```python
from build123d import *

# Parameters (mm, degrees)
SKETCH1_W               = 508
SKETCH1_H               = 228.6
BOSS_EXTRUDE1_DEPTH     = 254
SKETCH2_W               = 127
SKETCH2_H               = 93.154290468
CUT_EXTRUDE1_DEPTH      = 509
CUT_EXTRUDE2_DEPTH      = 254
SKETCH7_W               = 127
SKETCH7_H               = 101.6
CUT_EXTRUDE3_DEPTH      = 127
CUT_EXTRUDE5_DEPTH      = 127
CUT_EXTRUDE5_DEPTH_BACK = 0.254
SKETCH24_W              = 127
SKETCH24_H              = 101.6
BOSS_EXTRUDE3_DEPTH     = 63.5
CUT_EXTRUDE7_DEPTH      = 315.976
SKETCH27_R              = 6.604
CUT_EXTRUDE8_DEPTH      = 315.976


with BuildPart() as part:
    # Sketch1 → Boss-Extrude1 (new body)
    with BuildSketch(Plane.XY):
        Rectangle(SKETCH1_W, SKETCH1_H)
    extrude(amount=BOSS_EXTRUDE1_DEPTH)

    # Sketch2 → Cut-Extrude1 (cut, through all)
    with BuildSketch(Plane.ZY.offset(254)):
        with Locations((127, 67.722854766)):
            Rectangle(SKETCH2_W, SKETCH2_H)
    extrude(amount=-CUT_EXTRUDE1_DEPTH, mode=Mode.SUBTRACT)

    # Sketch5 → Cut-Extrude2 (cut)
    with BuildSketch(Plane.XY.offset(254)):
        Polygon((-254, 0), (-254, -114.3), (127, -114.3), (-63.5, 0), align=None)
    extrude(amount=-CUT_EXTRUDE2_DEPTH, mode=Mode.SUBTRACT)

    # Sketch7 → Cut-Extrude3 (cut)
    with BuildSketch(Plane(origin=(254, 0, 0), x_dir=(0, 0, -1), z_dir=(1, 0, 0))):
        with Locations((-127, -29.654290468)):
            Rectangle(SKETCH7_W, SKETCH7_H)
    extrude(amount=-CUT_EXTRUDE3_DEPTH, mode=Mode.SUBTRACT)

    # Sketch20 → Cut-Extrude5 (cut, two sides)
    with BuildSketch(Plane(origin=(0, 0, 190.5), x_dir=(-1, 0, 0), z_dir=(0, 0, -1))) as cut_extrude5_sk:
        Polygon((-127, 21.145709532), (39.624, 21.145709532), (-127, -80.454290468), align=None)
    extrude(amount=CUT_EXTRUDE5_DEPTH, mode=Mode.SUBTRACT)
    extrude(cut_extrude5_sk.sketch, amount=-CUT_EXTRUDE5_DEPTH_BACK, mode=Mode.SUBTRACT)

    # Sketch24 → Boss-Extrude3 (add)
    with BuildSketch(Plane(origin=(254, 0, 0), x_dir=(0, 0, -1), z_dir=(1, 0, 0))):
        with Locations((-127, -29.654290468)):
            Rectangle(SKETCH24_W, SKETCH24_H)
    extrude(amount=-BOSS_EXTRUDE3_DEPTH)

    # Sketch26 → Cut-Extrude7 (cut)
    with BuildSketch(Plane.XY.offset(254)):
        Polygon((254, 114.3), (-63.5, 114.3), (254, 0), align=None)
    extrude(amount=-CUT_EXTRUDE7_DEPTH, mode=Mode.SUBTRACT)

    # Sketch27 → Cut-Extrude8 (cut)
    with BuildSketch(Plane.XY.offset(254)):
        with Locations((-203.2, 57.15)):
            Circle(SKETCH27_R)
    extrude(amount=-CUT_EXTRUDE8_DEPTH, mode=Mode.SUBTRACT)


solid = part.part
```
Could you check a few things on this model? Use its own coordinates, in mm. A direction names the side the tool comes from. Round coordinates to 2 decimals unless told otherwise and drop trailing zeros. Loops run counter-clockwise (first coordinate to the right, second up) from the corner with the lowest first, then second, coordinate; pieces in that order, holes last.
Q1. For P1, Ø12, axis at y = -7.5, z = 166, coming from the -X side; P2, Ø2, axis at x = 82.5, z = 225, coming from the +Y side; P3, Ø12, axis at x = 57, y = -9, coming from the -Z side; P4, Ø5, axis at x = 193, z = 131.5, coming from the +Y side, each with a flat end and sliding along its axis, tell me the tip position at first contact or that it passes through.
Q2. Please list where these lines run through material, in increasing order: L1, parallel to Z at x = -158, y = 39; L2, parallel to Y at x = -203.2, z = 232.5; L3, parallel to Y at x = 155.5, z = 114.
Q3. I want a section at A-A (x = -203.2). Write out the boundary of the cut face in (y, z).
Q4. I want a section at D-D (y = -40). Write out the boundary of the cut face in (x, z), and give its area (3 significant figures).
Q5. Thinking about a two-plate mould opening in X: for faces 1 (the flat face through (-160, 114.3, 31)), 2 (the flat face through (198.86, 19.85, 128.78)), 3 (the flat face through (33.08, -57.95, 128.78)), 4 (the flat face through (159, -80.454, 128)), which applies, pulls with the +X half, pulls with the -X half, needs draft (parallel to the pull), parting line crosses it, or undercut?
Q6. I want a section at B-B (z = 72.5). Write out the boundary of the cut face in (x, y).
Q7. I want a section at C-C (y = 57.15). Write out the boundary of the cut face in (x, z).
Q8. On a 3-axis mill with a long thin cutter (end or side, diameter ignored), from which of +Z, -Z, +X, -X, +Y, -Y can I reach the whole of each face in a straight line? I mean faces 5 (the flat face through (-148, 21.146, 126)), 6 (the flat face through (-157, 0, 129)), 7 (the flat face through (190.5, -29, 128)). Say none if no direction works.
Answer below:
1. P1: stops at x = -61
1. P2: stops at y = 62.1
1. P3: stops at z = 0
1. P4: stops at y = 21.15
2. L1: z = 0 to 63.5, 190.5 to 254
2. L2: y = 0 to 50.55, 63.75 to 114.3
2. L3: y = -114.3 to -80.45
3. outline: (0, 0) - (50.55, 0) - (50.55, 63.5) - (21.15, 63.5) - (21.15, 190.5) - (50.55, 190.5) - (50.55, 254) - (0, 254) - close; (63.75, 0) - (114.3, 0) - (114.3, 63.5) - (63.75, 63.5) - close; (63.75, 190.5) - (114.3, 190.5) - (114.3, 254) - (63.75, 254) - close
4. outline: (3.17, 0) - (254, 0) - (254, 254) - (3.17, 254) - close; hole (60.65, 63.5) - (190.5, 63.5) - (190.5, 190.5) - (127, 190.5) - (127, 190.75) - (60.65, 190.75) - close
4. area: 47,200 mm2
5. face 1: needs draft
5. face 2: pulls with the +X half
5. face 3: pulls with the -X half
5. face 4: undercut
6. outline: (-254, 0) - (-63.5, 0) - (127, -114.3) - (254, -114.3) - (254, 0) - (195.26, 21.15) - (190.5, 21.15) - (190.5, -80.45) - (127, -80.45) - (-39.62, 21.15) - (-254, 21.15) - close
7. outline: (-254, 0) - (-209.8, 0) - (-209.8, 63.5) - (-254, 63.5) - close; (-254, 190.5) - (-209.8, 190.5) - (-209.8, 254) - (-254, 254) - close; (-196.6, 0) - (95.25, 0) - (95.25, 63.5) - (-196.6, 63.5) - close; (-196.6, 190.5) - (95.25, 190.5) - (95.25, 254) - (-196.6, 254) - close
8. face 5: +X, -X, +Y
8. face 6: +Z, -Z, -X, -Y
8. face 7: +Y
